The model under review builds one solid part; all positions refer to its coordinate system, in mm. A direction names the side the tool comes from. Coordinates: 2 decimals unless noted, no trailing zeros. Order: outer loops, then holes, each group sorted by start corner. A loop starts at its lowest first (then second) coordinate and runs counter-clockwise, first axis right, second up. Notation, with made-up numbers: (60.5, -18) -> (73.5, -18) arc R6 ccw to (73.5, -7) -> close; hole circle Ø3 at (-7, 37.5). An arc over 180 degrees is marked (long way). Put each result on its own line as item: value.
from build123d import *

# Parameters (mm, degrees)
BOSS_EXTRUDE1_DEPTH = 24.75
BOSS_EXTRUDE2_DEPTH = 3
CUT_EXTRUDE1_DEPTH  = 111.932129109
CUT_EXTRUDE2_DEPTH  = 109.046199668
FILLET1_R           = 6


with BuildPart() as part:
    # Sketch1 → Boss-Extrude1 (new, symmetric)
    with BuildSketch(Plane.XY):
        Polygon((44, 34), (56.5, 55.650635095), (100, 30.535898385), (100, 21.035898385), (100, 0), (90, 0), (90, 5), (44, 5), (6, 5), (0, 5), (0, 14.5), (6, 14.5), (44, 14.5), align=None)
    extrude(amount=BOSS_EXTRUDE1_DEPTH, both=True)

    # Sketch2 → Boss-Extrude2 (add)
    with BuildSketch(Plane(origin=(0, 14.5, 0), x_dir=(1, 0, 0), z_dir=(0, 1, 0))):
        with BuildLine():
            Line((31, 8.25), (31, -8.25))
            ThreePointArc((31, -8.25), (22, -17.25), (13, -8.25))
            Line((13, -8.25), (13, 8.25))
            ThreePointArc((13, 8.25), (22, 17.25), (31, 8.25))
        make_face()
        with BuildLine():
            Line((28, 8.25), (28, -8.25))
            ThreePointArc((28, -8.25), (22, -14.25), (16, -8.25))
            Line((16, -8.25), (16, 8.25))
            ThreePointArc((16, 8.25), (22, 14.25), (28, 8.25))
        make_face(mode=Mode.SUBTRACT)
    extrude(amount=BOSS_EXTRUDE2_DEPTH)

    # Sketch3 → Cut-Extrude1 (cut, through all)
    with BuildSketch(Plane(origin=(0, 14.5, 0), x_dir=(1, 0, 0), z_dir=(0, 1, 0))):
        with BuildLine():
            Line((28, -8.25), (28, 8.25))
            ThreePointArc((28, 8.25), (22, 14.25), (16, 8.25))
            Line((16, 8.25), (16, -8.25))
            ThreePointArc((16, -8.25), (22, -14.25), (28, -8.25))
        make_face()
    extrude(amount=-CUT_EXTRUDE1_DEPTH, mode=Mode.SUBTRACT)

    # Sketch4 → Cut-Extrude2 (cut, through all)
    with BuildSketch(Plane(origin=(18.277568136, -10.552558883, 0), x_dir=(0, 0, 1), z_dir=(-0.8660254037844386, 0.5000000000000001, 0))):
        Polygon((-12.5, 76.444863729), (12.5, 76.444863729), (17.118802154, 68.444863729), (-17.118802154, 68.444863729), align=None)
    extrude(amount=-CUT_EXTRUDE2_DEPTH, mode=Mode.SUBTRACT)

    # Fillet1
    fillet1_edges = [part.edges().sort_by_distance(p)[0] for p in [
        (0, 9.75, -24.75),
        (0, 9.75, 24.75),
    ]]
    fillet(fillet1_edges, radius=FILLET1_R)


solid = part.part
Item 1: For faces 1 (the flat face through (77.95, 38.71, 14.78)), 2 (the flat face through (31, 16, 0)), 3 (the flat face through (44, 5, 0)), list the 3-axis set-ups (+Z, -Z, +X, -X, +Y, -Y) from which the entire face can be reached by the end or side of a thin tool; tool diameter is ignored.
Answers below:
face 1: none
face 2: +Z, -Z, +Y
face 3: +Z, -Z, -X, -Y
Item 2: Consider section C-C on x = 92.5. Write out the cut boundary in (y, z).
Answers below:
outline: (0, -24.75) -> (34.87, -24.75) -> (34.87, -12.5) -> (25.63, -17.12) -> (25.63, 17.12) -> (34.87, 12.5) -> (34.87, 24.75) -> (0, 24.75) -> close
Item 3: Mouldability with a two-part tool opening along Z and no side actions: class faces 4 (the cylindrical face through (22.198, 15.979, 17.248)), 5 (the flat face through (64, 22, -24.75)), 6 (the cylindrical face through (21.87, 11.34, 14.25)), 7 (the cylindrical face through (22.13, 11.34, -14.25)) as +Z half, -Z half, draft (parallel to the pull), parting line (faces both ways), or undercut.
Answers below:
face 4: +Z half
face 5: -Z half
face 6: undercut
face 7: undercut
Item 4: For line 1 (X direction, y = 16.5, z = -13.5); line 2 (Y direction, x = 27, z = -20.5); line 3 (Y direction, x = 78, z = -9), list the stretches that pass through material, from the lowest coordinate up. Write a range as from..to.
Answers below:
line 1: 14.69..19.1, 24.9..29.31, 44..100
line 2: 5..14.5
line 3: 5..34
Item 5: Consider section A-A on z = -2. Write out the cut boundary in (x, y).
Answers below:
outline: (0, 5) -> (16, 5) -> (16, 17.5) -> (13, 17.5) -> (13, 14.5) -> (0, 14.5) -> close; (28, 5) -> (90, 5) -> (90, 0) -> (100, 0) -> (100, 21.3) -> (52.5, 48.72) -> (44, 34) -> (44, 14.5) -> (31, 14.5) -> (31, 17.5) -> (28, 17.5) -> close
Item 6: Consider section B-B on x = 22. Write out the cut boundary in (y, z).
Answers below:
outline: (5, -24.75) -> (14.5, -24.75) -> (14.5, -17.25) -> (17.5, -17.25) -> (17.5, -14.25) -> (5, -14.25) -> close; (5, 14.25) -> (17.5, 14.25) -> (17.5, 17.25) -> (14.5, 17.25) -> (14.5, 24.75) -> (5, 24.75) -> close
Item 7: For pin 1 Ø12 at (x, y) = (44, 45.5) entering from -Z; pin 2 Ø3 at (x, z) = (24.5, -11) entering from +Y; pin 3 Ø20 at (x, z) = (18, -3) entering from +Y; pin 4 Ø4 at (y, z) = (26, 11.5) entering from -X, all flat-tipped, find the tip position at first contact; note any pin that passes through.
Answers below:
pin 1: z = -24.75
pin 2: through
pin 3: y = 17.5
pin 4: x = 44
Item 8: Consider section D-D on y = 24. Write out the cut boundary in (x, z), and give its area (3 significant figures).
Answers below:
outline: (44, -24.75) -> (100, -24.75) -> (100, -15.77) -> (95.32, -17.12) -> (95.32, 17.12) -> (100, 15.77) -> (100, 24.75) -> (44, 24.75) -> close
area: 2,620 mm^2
